Print and shaded views of the part. All mm, measured from the part's lowest x, y and z. Coordinates: 2 decimals unless noted, no trailing zeros. Loops run counter-clockwise (first coordinate to the right, second up) from the corner with the lowest first, then second, coordinate; pieces in that order, holes last. Notation, with made-up numbers: (-12.5, 87) -> (26.5, 87) arc R34 cw to (26.5, 125) -> close; hole circle Ø8 at (31.25, 10.25). An arc over 180 degrees is marked (long way). One line per question, with ' | ' between items. Start each with the question number.
1) Probe L1, parallel to X at y = 74.5, z = 1.7 (1 decimal); L2, parallel to X at y = 46, z = 0.65 (1 decimal); L3, parallel to Y at x = 369, z = 0.9 (1 decimal). List the from-to ranges inside material, lowest first. Write a range as from..to.
2) Cut at B-B (y = 40.8). List the corners of the cut face in (x, z) (1 decimal), plus the area to 3 significant figures.
3) Cut at C-C (x = 40.8). List the corners of the cut face in (y, z) (1 decimal).
4) Cut at D-D (y = 22). List the corners of the cut face in (x, z) (1 decimal), plus the area to 3 significant figures.
5) Cut at A-A (z = 1.45). List the corners of the cut face in (x, y) (1 decimal).
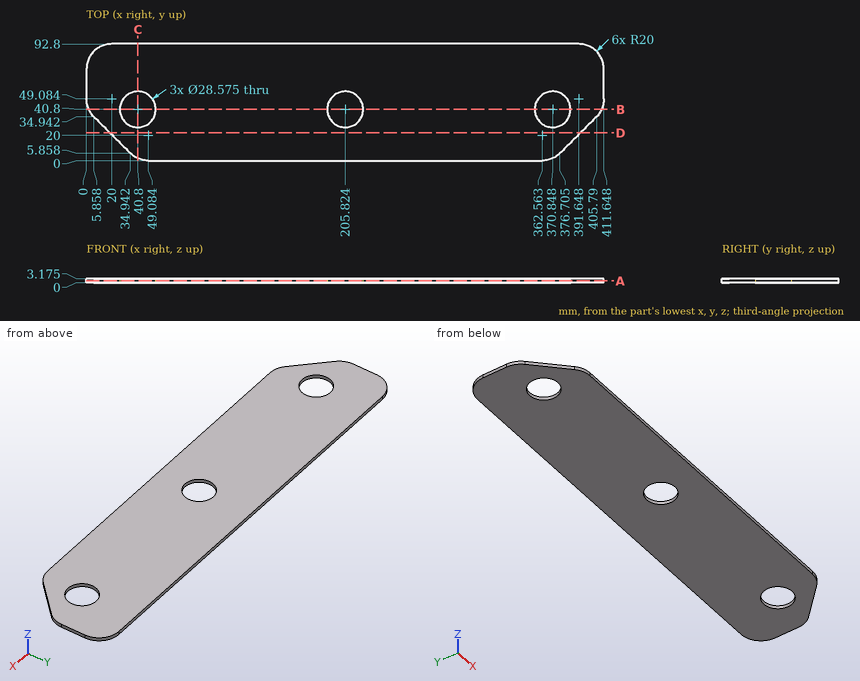
Reported:
1) L1: x = 0.1..411.6 | L2: x = 0.2..27.5, 54.1..192.5, 219.1..357.5, 384.2..411.4 | L3: y = 1.1..26.6, 55..92.8
2) outline: (1.8, 0) -> (26.5, 0) -> (26.5, 3.2) -> (1.8, 3.2) -> close; (55.1, 0) -> (191.5, 0) -> (191.5, 3.2) -> (55.1, 3.2) -> close; (220.1, 0) -> (356.6, 0) -> (356.6, 3.2) -> (220.1, 3.2) -> close; (385.1, 0) -> (409.9, 0) -> (409.9, 3.2) -> (385.1, 3.2) -> close | area: 1,020 mm²
3) outline: (1.8, 0) -> (26.5, 0) -> (26.5, 3.2) -> (1.8, 3.2) -> close; (55.1, 0) -> (92.8, 0) -> (92.8, 3.2) -> (55.1, 3.2) -> close
4) outline: (18.8, 0) -> (392.8, 0) -> (392.8, 3.2) -> (18.8, 3.2) -> close | area: 1,190 mm²
5) outline: (0, 49.1) arc R20 ccw to (5.9, 34.9) -> (34.9, 5.9) arc R20 ccw to (49.1, 0) -> (362.6, 0) arc R20 ccw to (376.7, 5.9) -> (405.8, 34.9) arc R20 ccw to (411.6, 49.1) -> (411.6, 72.8) arc R20 ccw to (391.6, 92.8) -> (20, 92.8) arc R20 ccw to (0, 72.8) -> close; hole circle Ø28.6 at (40.8, 40.8); hole circle Ø28.6 at (205.8, 40.8); hole circle Ø28.6 at (370.8, 40.8)
